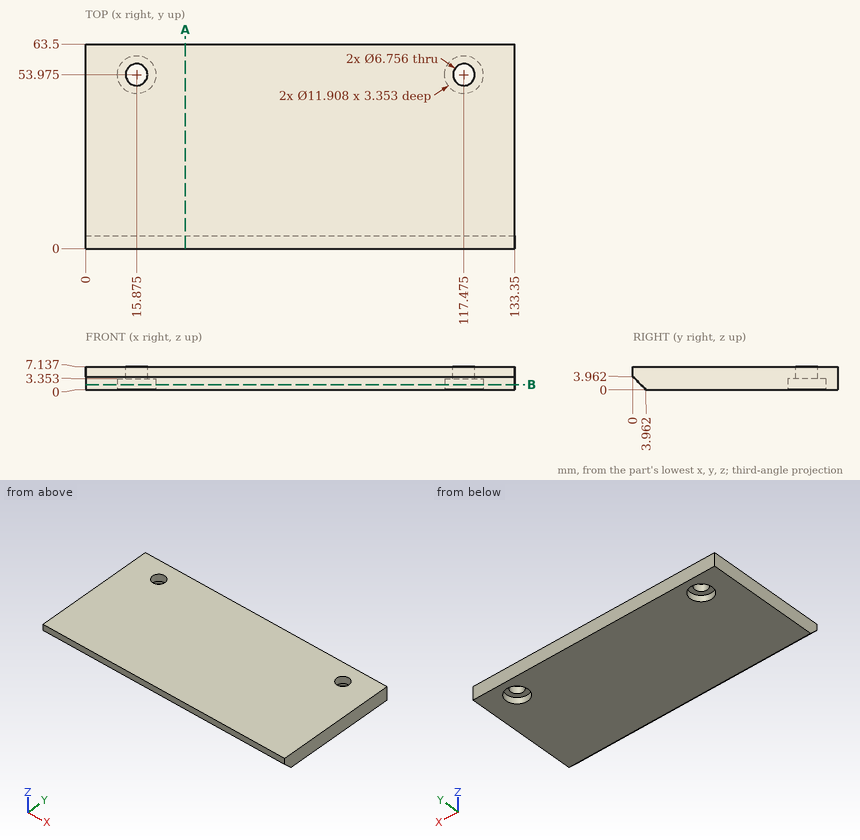
Print and shaded views of the part. All mm, measured from the part's lowest x, y and z. Coordinates: 2 decimals unless noted, no trailing zeros. Write each loop counter-clockwise with the first axis right and the second up, starting at its lowest first coordinate (ties: lowest second). Pieces come first, ordered by that corner, then holes. Notation, with made-up numbers: M 33.5,-16.75 L 39.5,-16.75 A25 ccw 39.5,10.25 Z; hole C -0.5,-33 d11. An arc over 180 degrees is marked long. Return JSON: item names as keys, results as strings.
1. Saw through at B-B, the plane z = 1.5. Count the separate pieces of the cut face and the enclosed holes in it, then the cut area to 3 significant figures.
Determined:
{"separate pieces": "1", "enclosed holes": "2", "area": "7,920 mm²"}
2. Probe L1, parallel to Y at x = 117.5, z = 6.25; L2, parallel to Y at x = 21, z = 1 (1 decimal); L3, parallel to Z at x = 112.5, y = 53. List the from-to ranges inside material, lowest first.
Determined:
{"L1": "0 to 50.6, 57.35 to 63.5", "L2": "3 to 50.9, 57 to 63.5", "L3": "3.35 to 7.14"}
3. Flat gauge pin, fed straight in: pin 1 Ø10.5 at (x, y) = (117.475, 53.975) entering from -Z. Where does the tip first touch, or does it go through?
Determined:
{"pin 1": "z = 3.35"}
4. Saw through at A-A, the plane x = 31. Write the cut outline in (y, z).
Determined:
{"outline": "M 0,3.96 L 3.96,0 L 63.5,0 L 63.5,7.14 L 0,7.14 Z"}
